For this review, take the finished solid that the model builds, in its own axes (mm). A direction names the side the tool comes from. Round coordinates to 2 decimals unless told otherwise and drop trailing zeros. Loops run counter-clockwise (first coordinate to the right, second up) from the corner with the lowest first, then second, coordinate; pieces in that order, holes last. Notation, with made-up numbers: M -24,53 L 31,53 A14 ccw 31,71 Z; hole C -15.75,2 d5. An arc over 180 degrees is marked long. Write item = value, one per line. Start each with the question number.
```python
from build123d import *

# Parameters (mm, degrees)
F0_W     = 59.5000050962
F0_H     = 32.5015373528
F1_DEPTH = 25
F2_W     = 59.5000050962
F2_H     = 32.5015373528
F3_DEPTH = 20
F4_SIZE  = 15
F5_W     = 10.4703865945
F5_H     = 18.7411587685
F5_W_2   = 13.4615413845
F5_H_2   = 8.076922968
F6_DEPTH = 5
F7_W     = 8.1467057019
F7_H     = 2.5015373528
F8_DEPTH = 5


with BuildPart() as f1:
    # F0 (on Top) → F1 (new body)
    with BuildSketch(Plane.XY):
        with Locations((29.7500025481, 16.2507686764)):
            Rectangle(F0_W, F0_H)
    extrude(amount=F1_DEPTH)

    # F2 (on face) → F3 (join)
    with BuildSketch(Plane.XY.offset(25)):
        with Locations((29.7500025481, 16.2507686764)):
            Rectangle(F2_W, F2_H)
    extrude(amount=F3_DEPTH)

    # F4
    f4_edges = [f1.edges().sort_by_distance(p)[0] for p in [
        (0, 16.250769, 45),
        (59.500005, 16.250769, 45),
        (29.750003, 0, 45),
        (29.750003, 32.501537, 45),
    ]]
    chamfer(f4_edges, length=F4_SIZE)

    # F5 (on face) → F6 (cut)
    with BuildSketch(Plane.XZ):
        with Locations((14.1790322959, 9.3705793843)):
            Rectangle(F5_W, F5_H)
        with Locations((35.4199837893, 14.7026972845)):
            Rectangle(F5_W_2, F5_H_2)
    extrude(amount=-F6_DEPTH, mode=Mode.SUBTRACT)

    # F7 (on face) → F8 (join)
    with BuildSketch(Plane.XY.offset(45)):
        with Locations((19.073352851, 16.2507686764)):
            Rectangle(F7_W, F7_H)
    extrude(amount=F8_DEPTH)


solid = f1.part
```
(1) Add section D-D on z = 18. Write out the cut boundary in (x, y).
(2) For pin 1 Ø2.5 at (x, z) = (17.5, 47.5) entering from +Y; pin 2 Ø9 at (x, z) = (37, 15.5) entering from -Y; pin 3 Ø4 at (x, y) = (41.5, 11.5) entering from +Z; pin 4 Ø1.5 at (x, y) = (35.5, 2.5) entering from +Z, all flat-tipped, find the tip position at first contact; note any pin that passes through.
(3) Draft analysis for pull direction Z (two halves, no side actions). For faces 5 (the flat face through (19, 16, 50)), 6 (the flat face through (19, 15, 47)), 7 (the flat face through (35, 2, 18.741)), state which applies: +Z half, -Z half, draft (parallel to the pull), parting line (faces both ways), or undercut.
(4) Wall thickness on L1, parallel to Y at x = 37, z = 12; L2, parallel to Z at x = 38, y = 4; L3, parallel to Z at x = 11.5, y = 18: over which ranges is each line inside the solid? List them lowest first.
(5) Add section A-A on z = 7.5. Write out the cut boundary in (x, y), and give its area (3 significant figures).
(6) Tool access review of faces 1 (the flat face through (14, 2, 18.741)), 2 (the flat face through (23.147, 16, 47)), 3 (the flat face through (28.689, 2, 15)), 4 (the flat face through (19, 17.502, 47)): name each direction out of +Z, -Z, +X, -X, +Y, -Y from which nothing blocks a thin tool from reaching the whole face with its end or side.
(7) Add section B-B on x = 18. Write out the cut boundary in (y, z).
(8) Add section C-C on y = 14. Write out the cut boundary in (x, z).
Answer sheet:
q1.outline = M 0,0 L 8.94,0 L 8.94,5 L 19.41,5 L 19.41,0 L 28.69,0 L 28.69,5 L 42.15,5 L 42.15,0 L 59.5,0 L 59.5,32.5 L 0,32.5 Z
q2.pin_1 = 17.5
q2.pin_2 = 0
q2.pin_3 = 43.5
q2.pin_4 = 33.25
q3.face_5 = +Z half
q3.face_6 = draft
q3.face_7 = undercut
q4.L1 = 5 to 32.5
q4.L2 = 0 to 10.66, 18.74 to 34
q4.L3 = 0 to 41.5
q5.outline = M 0,0 L 8.94,0 L 8.94,5 L 19.41,5 L 19.41,0 L 59.5,0 L 59.5,32.5 L 0,32.5 Z
q5.area = 1,880 mm²
q6.face_1 = -Z, -Y
q6.face_2 = +Z, +X, +Y, -Y
q6.face_3 = -Y
q6.face_4 = +Z, +X, -X, +Y
q7.outline = M 0,18.74 L 5,18.74 L 5,0 L 32.5,0 L 32.5,30 L 17.5,45 L 17.5,50 L 15,50 L 15,45 L 0,30 Z
q8.outline = M 0,0 L 59.5,0 L 59.5,30 L 45.5,44 L 14,44 L 0,30 Z
